from build123d import *

# Parameters (mm, degrees)
SKETCH1_R                   = 60
MAIN_EXTRUDE_DEPTH          = 260
SKETCH2_R                   = 56
HOLE_FOR_BLADE_CASING_DEPTH = 40
HOLE_START                  = -20
SKETCH3_R                   = 56
HOLE_TO_HIDE_LEGS_DEPTH     = 20
LIGHTNING_BOLT_REACH        = 296.575
LIGHTNING_BOLT_START_RADIUS = 60
LIGHTNING_BOLT_END_RADIUS   = 60
SKETCH5_R                   = 16
LEGS_DEPTH                  = 19


with BuildPart() as part:
    # Sketch1 → Main Extrude (new body)
    with BuildSketch(Plane(origin=(0, 0, 0), x_dir=(1, 0, 0), z_dir=(0, 1, 0))):
        with Locations(Location((0, 0, 0), (0, 0, 270))):
            Circle(SKETCH1_R)
    extrude(amount=MAIN_EXTRUDE_DEPTH)

    # Sketch2 → Hole for Blade Casing (cut)
    with BuildSketch(Plane(origin=(0, 260, 0), x_dir=(1, 0, 0), z_dir=(0, 1, 0))):
        with Locations(Location((0, 0, 0), (0, 0, 270))):
            Circle(SKETCH2_R)
    extrude(amount=-HOLE_FOR_BLADE_CASING_DEPTH, mode=Mode.SUBTRACT)

    # Sketch3 → Hole to Hide Legs (cut)
    with BuildSketch(Plane.XZ.offset(HOLE_START)):
        with Locations(Location((0, 0, 0), (0, 0, 90))):
            Circle(SKETCH3_R)
    extrude(amount=HOLE_TO_HIDE_LEGS_DEPTH, mode=Mode.SUBTRACT)

    # Lightning Bolt: from a cylinder face, 296.575 long prism both ways, kept between that surface and its translate by the depth
    lightning_bolt_start = Plane(origin=(0, 160, 0), z_dir=(0, -1, 0)) * Cylinder(LIGHTNING_BOLT_START_RADIUS, 714.15, mode=Mode.PRIVATE)
    lightning_bolt_end = Plane(origin=(0, 160, -2), z_dir=(0, -1, 0)) * Cylinder(LIGHTNING_BOLT_END_RADIUS, 714.15, mode=Mode.PRIVATE)
    # Sketch4 → Lightning Bolt (cut, from a surface)
    with BuildSketch(Plane.XY.offset(60), mode=Mode.PRIVATE) as lightning_bolt_sk1:
        Polygon((0, 220), (-40, 160), (0, 140), (0, 100), (40, 160), (0, 180), align=None)
    lightning_bolt_tool1 = extrude(lightning_bolt_sk1.sketch, amount=LIGHTNING_BOLT_REACH, both=True, mode=Mode.PRIVATE)
    add(((lightning_bolt_tool1 & lightning_bolt_start) - lightning_bolt_end).solids().sort_by_distance((0, 160, 51.36068))[0], mode=Mode.SUBTRACT)

    # Sketch5 → Legs (add)
    with BuildSketch(Plane.XZ.offset(-20)):
        with Locations(Location((-24.748737342, 24.748737342, 0), (0, 0, 270))):
            Circle(SKETCH5_R)
        with Locations(Location((24.748737342, 24.748737342, 0), (0, 0, 270))):
            Circle(SKETCH5_R)
        with Locations(Location((24.748737342, -24.748737342, 0), (0, 0, 270))):
            Circle(SKETCH5_R)
        with Locations(Location((-24.748737342, -24.748737342, 0), (0, 0, 270))):
            Circle(SKETCH5_R)
    extrude(amount=LEGS_DEPTH)


solid = part.part
Input: part model. Units: mm. Frame: model coordinates. A direction names the side the tool comes from. Coordinates: 2 decimals unless noted, no trailing zeros. Loops run counter-clockwise (first coordinate to the right, second up) from the corner with the lowest first, then second, coordinate; pieces in that order, holes last.
(1) Section D-D on y = 43.5. Return the cut outline in (x, z), then the cut area to 3 significant figures.
(2) Pull-direction query (X, two-part tool) for faces 1 (the face through (2.64, 128.18, -59.94)), 2 (the face through (-40, 0, 40)), 3 (the face through (25, 1, -25)); classes: released by +X, released by -X, zero draft, split by the parting line, or undercut.
(3) Material intervals for probe 1 along X at (y, z) = (13.5, 0); probe 2 along Y at (x, z) = (21, -49.5); probe 3 along Z at (x, y) = (26, 221.5), sorted ascending.
(4) Section B-B on x = 49. Return the cut outline in (y, z).
(5) Set-up query: faces 4 (the face through (-38.943, 10.633, -32.132)), 5 (the face through (1, 220, -1)), 6 (the face through (-40, 260, 40)). Return all of +Z, -Z, +X, -X, +Y, -Y with unobstructed straight access to the full face (end or side cutting, diameter ignored); none if empty.
(6) Section C-C on y = 227.5. Return the cut outline in (x, z), then the cut area to 3 significant figures.
(7) Section A-A on z = 0. Return the cut outline in (x, y).
(8) First-contact query: pin 1 Ø1.5 at (x, z) = (-9.5, -40.5) entering from +Y; pin 2 Ø8 at (x, z) = (32, 8.5) entering from -Y; pin 3 Ø1 at (x, z) = (-43.5, -9.5) entering from -Y. Flat tips, straight axial feed; report the tip coordinate or a pass-through.
Data:
1. outline: circle Ø120 at (0, 0)
1. area: 11,300 mm2
2. face 1: split by the parting line
2. face 2: zero draft
2. face 3: undercut
3. probe 1: x = -60 to -56, 56 to 60
3. probe 2: y = 20 to 220
3. probe 3: z = -54.07 to -49.6, 49.6 to 54.07
4. outline: (0, -34.63) - (260, -34.63) - (260, -27.11) - (220, -27.11) - (220, 27.11) - (260, 27.11) - (260, 34.63) - (0, 34.63) - (0, 27.11) - (20, 27.11) - (20, -27.11) - (0, -27.11) - close
5. face 4: -Y
5. face 5: +Y
5. face 6: +Z, -Z, +X, -X, +Y
6. outline: circle Ø120 at (0, 0); hole circle Ø112 at (0, 0)
6. area: 1,460 mm2
7. outline: (-60, 0) - (-56, 0) - (-56, 20) - (56, 20) - (56, 0) - (60, 0) - (60, 260) - (56, 260) - (56, 220) - (-56, 220) - (-56, 260) - (-60, 260) - close
8. pin 1: stops at y = 220
8. pin 2: stops at y = 1
8. pin 3: stops at y = 20
